The listing builds one solid part. Answer for the finished solid, in the listing's coordinates (mm). A direction names the side the tool comes from. Round coordinates to 2 decimals unless told otherwise and drop trailing zeros. Loops run counter-clockwise (first coordinate to the right, second up) from the corner with the lowest first, then second, coordinate; pieces in that order, holes last. Notation, with made-up numbers: M 52,17 L 70,17 A29 cw 70,38 Z; hole C 61.5,-22.75 d7. An arc over 180 degrees is marked long. Put each result on its own line as item: value. Start each with the question number.
(1) Section C-C, the plane z = 1.4 is taken. Determine the outline of the cut face in (x, y).
(2) Which of the six approach directions +Z, -Z, +X, -X, +Y, -Y give full straight-line access (tool end or side, diameter ignored) to faces 5 (the face through (48, 39, 2)), 6 (the face through (35.35, -25, 1))?
(3) A flat-ended cylindrical pin translates along its axis: P1, Ø16, axis at x = -8.5, y = 25, coming from the -Z side. Find the tip coordinate at first contact, or state that the pin passes through.
(4) Straight lines are drawn through the part: line 1 (Y direction, x = 9.5, z = 0.45); line 2 (Y direction, x = -39.85, z = 1.9); line 3 (X direction, y = -34, z = 1.95). For each, find the intervals that lie inside material, in ascending order.
(5) Section B-B, the plane x = -39.85 is taken. Determine the outline of the cut face in (y, z).
(6) Determine the mould class of faces 1 (the face through (50, 0, 1)), 2 (the face through (-1, -40, 1)), 3 (the face through (0, -25, 2)), 4 (the face through (-49, -38, 2)) for opening direction X: released by +X, released by -X, zero draft, split by the parting line, or undercut.
(7) Section D-D, the plane y = 31.5 is taken. Determine the outline of the cut face in (x, z), then the cut area to 3 significant figures.
(8) Section A-A, the plane y = 22.85 is taken. Determine the outline of the cut face in (x, z), then the cut area to 3 significant figures.
```python
from build123d import *

# Parameters (mm, degrees)
SKETCH_W     = 100
SKETCH_H     = 80
SKETCH_R     = 1.35
PAD_DEPTH    = 3
SKETCH001_W  = 70.7
SKETCH001_H  = 20.2
POCKET_DEPTH = 2
FILLET_R     = 5


with BuildPart() as part:
    # Sketch → Pad (new body)
    with BuildSketch(Plane.XY):
        Rectangle(SKETCH_W, SKETCH_H)
        with Locations((-39.85, 22.85)):
            Circle(SKETCH_R, mode=Mode.SUBTRACT)
        with Locations((45.95, 22.85)):
            Circle(SKETCH_R, mode=Mode.SUBTRACT)
        with Locations((-39.85, -35.95)):
            Circle(SKETCH_R, mode=Mode.SUBTRACT)
        with Locations((45.95, -35.95)):
            Circle(SKETCH_R, mode=Mode.SUBTRACT)
    extrude(amount=PAD_DEPTH)

    # Sketch001 (on Face9 of Pad) → Pocket (cut)
    with BuildSketch(Plane(origin=(0, 0, 0), x_dir=(1, 0, 0), z_dir=(0, 0, -1))):
        with Locations((0, 24.9)):
            Rectangle(SKETCH001_W, SKETCH001_H)
        with Locations((0, -24.9)):
            Rectangle(SKETCH001_W, SKETCH001_H)
    extrude(amount=-POCKET_DEPTH, mode=Mode.SUBTRACT)

    # Fillet
    fillet_edges = [part.edges().sort_by_distance(p)[0] for p in [
        (-50, 40, 1.5),
        (50, 40, 1.5),
        (-50, -40, 1.5),
        (50, -40, 1.5),
    ]]
    fillet(fillet_edges, radius=FILLET_R)


solid = part.part
```
Recorded:
1. outline: M -50,-35 A5 ccw -45,-40 L 45,-40 A5 ccw 50,-35 L 50,35 A5 ccw 45,40 L -45,40 A5 ccw -50,35 Z; hole C -39.85,-35.95 d2.7; hole C -39.85,22.85 d2.7; hole M -35.35,-35 L 35.35,-35 L 35.35,-14.8 L -35.35,-14.8 Z; hole M -35.35,14.8 L 35.35,14.8 L 35.35,35 L -35.35,35 Z; hole C 45.95,-35.95 d2.7; hole C 45.95,22.85 d2.7
2. face 5: +Z, -Z, +X, +Y
2. face 6: -Z
3. P1: stops at z = 2
4. line 1: y = -40 to -35, -14.8 to 14.8, 35 to 40
4. line 2: y = -40 to -37.3, -34.6 to 21.5, 24.2 to 40
4. line 3: x = -50 to -35.35, 35.35 to 50
5. outline: M -40,0 L -37.3,0 L -37.3,3 L -40,3 Z; M -34.6,0 L 21.5,0 L 21.5,3 L -34.6,3 Z; M 24.2,0 L 40,0 L 40,3 L 24.2,3 Z
6. face 1: released by +X
6. face 2: zero draft
6. face 3: undercut
6. face 4: released by -X
7. outline: M -50,0 L -35.35,0 L -35.35,2 L 35.35,2 L 35.35,0 L 50,0 L 50,3 L -50,3 Z
7. area: 159 mm²
8. outline: M -50,0 L -41.2,0 L -41.2,3 L -50,3 Z; M -38.5,0 L -35.35,0 L -35.35,2 L 35.35,2 L 35.35,0 L 44.6,0 L 44.6,3 L -38.5,3 Z; M 47.3,0 L 50,0 L 50,3 L 47.3,3 Z
8. area: 142 mm²
